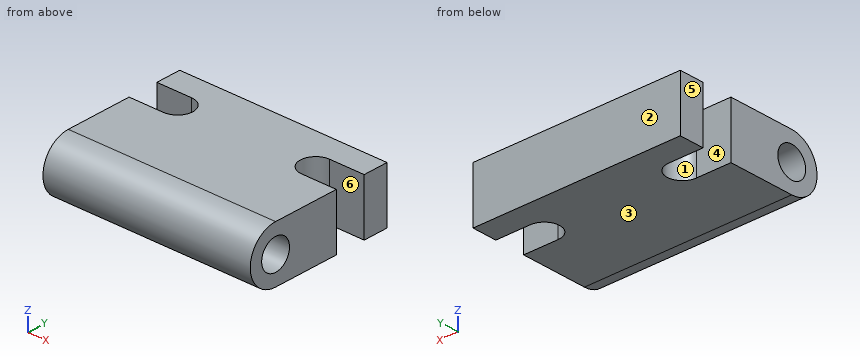
from build123d import *

# Parameters (mm, degrees)
F0_R     = 11
F1_DEPTH = 150
F3_DEPTH = 50


with BuildPart() as f1:
    # F0 (on Right) → F1 (new body)
    with BuildSketch(Plane.YZ):
        with BuildLine():
            Line((44, 40), (-44, 40))
            ThreePointArc((-44, 40), (-64, 20), (-44, 0))
            Line((-44, 0), (44, 0))
            Line((44, 0), (44, 40))
        make_face()
        with Locations((-44, 20)):
            Circle(F0_R, mode=Mode.SUBTRACT)
    extrude(amount=F1_DEPTH)

    # F2 (on face) → F3 (cut)
    with BuildSketch(Plane.XY.offset(40)):
        with BuildLine():
            Line((150, 4), (150, 26))
            Line((150, 26), (125, 26))
            ThreePointArc((125, 26), (114, 15), (125, 4))
            Line((125, 4), (150, 4))
        make_face()
        with BuildLine():
            Line((25, 26), (0, 26))
            Line((0, 26), (0, 4))
            Line((0, 4), (25, 4))
            ThreePointArc((25, 4), (36, 15), (25, 26))
        make_face()
    extrude(amount=-F3_DEPTH, mode=Mode.SUBTRACT)


solid = f1.part
The model under review builds one solid part; all positions refer to its coordinate system, in mm. Face numbers are marked on the shaded views. A direction names the side the tool comes from. Coordinates: 2 decimals unless noted, no trailing zeros. Loops run counter-clockwise (first coordinate to the right, second up) from the corner with the lowest first, then second, coordinate; pieces in that order, holes last. Notation, with made-up numbers: (-34, 28.5) -> (6, 28.5) arc R10 cw to (6, 46.5) -> close; hole circle Ø3 at (-27.5, 22). An arc over 180 degrees is marked (long way). Use a Markdown table: item, result. Add a question column.
1. Add section C-C on x = 62. Write out the cut boundary in (y, z), plus the area to 3 significant figures.
2. Add section D-D on y = -37.5. Write out the cut boundary in (x, z).
3. Machinability: for the marked faces 4, 5 and 6, which of the approach directions +Z, -Z, +X, -X, +Y, -Y give a long, thin tool a straight path to every point of the face, cutting with its end or side? Answer none if there is none.
4. Clearance check with flat-ended pins moving along their axes: pin 1 Ø8 at (x, y) = (86.5, -52) entering from +Z; pin 2 Ø3 at (x, z) = (60.5, 32) entering from -Y; pin 3 Ø4 at (x, z) = (85, 13.5) entering from -Y. State where each tip first meets the part, or that it passes through.
5. Add section B-B on z = 20. Write out the cut boundary in (x, y), plus the area to 3 significant figures.
6. To check wall thickness, follow line 1 (Y direction, x = 12, z = 15.5); line 2 (Z direction, x = 59.5, y = -44); line 3 (Y direction, x = 117, z = 7). State the ranges of each line that lie inside material, in increasing order.
7. Add section A-A on x = 21. Write out the cut boundary in (y, z).
8. Draft analysis for pull direction Y (two halves, no side actions). For the marked faces 1, 2 and 3, state which applies: pulls with the +Y half, pulls with the -Y half, needs draft (parallel to the pull), parting line crosses it, or undercut.
Returned:
| question | item | result |
|---|---|---|
| 1 | outline | (-44, 0) -> (44, 0) -> (44, 40) -> (-44, 40) arc R20 ccw to start; hole circle Ø22 at (-44, 20) |
| 1 | area | 3,770 mm² |
| 2 | outline | (0, 0) -> (150, 0) -> (150, 11.13) -> (0, 11.13) -> close; (0, 28.87) -> (150, 28.87) -> (150, 40) -> (0, 40) -> close |
| 3 | face 4 | +Z, -Z, -X |
| 3 | face 5 | +Z, -Z, -X, +Y, -Y |
| 3 | face 6 | +Z, -Z, +X |
| 4 | pin 1 | stops at z = 39.6 |
| 4 | pin 2 | stops at y = -61.02 |
| 4 | pin 3 | stops at y = -63.49 |
| 5 | outline | (0, -64) -> (150, -64) -> (150, -55) -> (0, -55) -> close; (0, -33) -> (150, -33) -> (150, 4) -> (125, 4) arc R11 cw to (125, 26) -> (150, 26) -> (150, 44) -> (0, 44) -> (0, 26) -> (25, 26) arc R11 cw to (25, 4) -> (0, 4) -> close |
| 5 | area | 11,400 mm² |
| 6 | line 1 | y = -63.49 to -54.04, -33.96 to 4, 26 to 44 |
| 6 | line 2 | z = 0 to 9, 31 to 40 |
| 6 | line 3 | y = -59.2 to 7.45, 22.55 to 44 |
| 7 | outline | (-44, 0) -> (4, 0) -> (4, 40) -> (-44, 40) arc R20 ccw to start; (26, 0) -> (44, 0) -> (44, 40) -> (26, 40) -> close; hole circle Ø22 at (-44, 20) |
| 8 | face 1 | undercut |
| 8 | face 2 | pulls with the +Y half |
| 8 | face 3 | needs draft |
